from build123d import *

# Parameters (mm, degrees)
BOSS_EXTRUDE1_DEPTH = 2
SCALE1_SCALE        = 0.6


with BuildPart() as part:
    # Sketch1 → Boss-Extrude1 (new body)
    with BuildSketch(Plane.XY):
        with BuildLine():
            Line((-87.945199987, 16.915862102), (-85.508172497, 19.844172117))
            Line((-85.508172497, 19.844172117), (51.705430776, 19.844172117))
            Line((51.705430776, 19.844172117), (54.142458266, 16.915862102))
            ThreePointArc((54.142458266, 16.915862102), (68.102505257, 0), (54.142458266, -16.915862102))
            Line((54.142458266, -16.915862102), (51.705430776, -19.844172117))
            Line((51.705430776, -19.844172117), (-85.508172497, -19.844172117))
            Line((-85.508172497, -19.844172117), (-87.945199987, -16.915862102))
            ThreePointArc((-87.945199987, -16.915862102), (-101.800450477, -0.05365779), (-88.010047693, 16.861622033))
            ThreePointArc((-88.010047693, 16.861622033), (-87.975174361, 16.885813548), (-87.945199987, 16.915862102))
        make_face()
    extrude(amount=BOSS_EXTRUDE1_DEPTH)


with BuildPart() as part_1:
    # Scale1: scaled about (-16.855793262, -0.001137482, 1)
    add(part.part.scale(SCALE1_SCALE).moved(Location((-6.742317305, -0.000454993, 0.4))))


solid = part_1.part
Geometry: final body of the model. Coordinates: model frame, mm. Give positions to 0.01 mm unless a question says otherwise; leave off trailing zeros. Write each loop counter-clockwise with the first axis right and the second up, starting at its lowest first coordinate (ties: lowest second). Pieces come first, ordered by that corner, then holes. Notation, with made-up numbers: M 2.25,88.25 L 9.25,88.25 A11 cw 9.25,95.25 Z; hole C 70.5,-26.5 d7. An arc over 180 degrees is marked long. Answer in a Markdown table with one row per item. Add a question column.
(1) Section B-B on y = -6.25. Return loops of the section in (x, z), and give its area (3 significant figures).
(2) Ray query, line 1 (X direction, y = 0.25, z = 0.8); line 2 (X direction, y = 5.75, z = 1.4). Return the intervals inside material, ascending.
(3) Section A-A on z = 1.35. Return loops of the section in (x, y), and give its area (3 significant figures).
(4) Section C-C on y = 7.5. Return loops of the section in (x, z).
Result set:
| question | item | result |
|---|---|---|
| 1 | outline | M -65.73,0.4 L 32.02,0.4 L 32.02,1.6 L -65.73,1.6 Z |
| 1 | area | 117 mm^2 |
| 2 | line 1 | x = -67.82 to 34.12 |
| 2 | line 2 | x = -66.07 to 32.37 |
| 3 | outline | M -59.55,10.12 A10.34 ccw -59.51,-10.15 L -58.05,-11.91 L 24.28,-11.91 L 25.74,-10.15 A10.34 ccw 25.74,10.15 L 24.28,11.91 L -58.05,11.91 L -59.51,10.15 A0.14 cw Z |
| 3 | area | 2,280 mm^2 |
| 4 | outline | M -64.59,0.4 L 30.9,0.4 L 30.9,1.6 L -64.59,1.6 Z |
